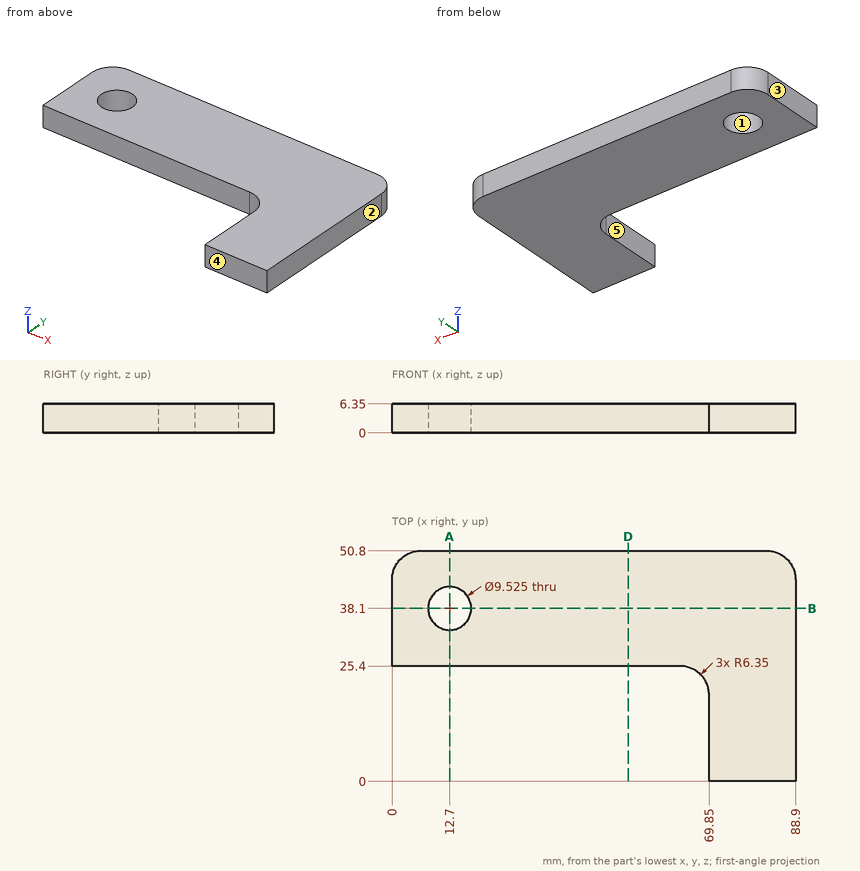
For this review, use the dimensioned drawing (mm, ordinates from the lowest corner) and the shaded views. A direction names the side the tool comes from. Give positions to 0.01 mm unless a question says otherwise; leave off trailing zeros. Loops run counter-clockwise (first coordinate to the right, second up) from the corner with the lowest first, then second, coordinate; pieces in that order, holes last. Notation, with made-up numbers: (-2, 36) -> (23, 36) arc R18 ccw to (23, 52) -> close; hole circle Ø7 at (64.25, 31.5). An arc over 180 degrees is marked (long way). One line per question, with ' | ' between items. Start each with the question number.
(1) For the marked faces 4 and 5, list the 3-axis set-ups (+Z, -Z, +X, -X, +Y, -Y) from which the entire face can be reached by the end or side of a thin tool; tool diameter is ignored.
(2) We need section D-D (x = 52). State the section outline as (y, z) points.
(3) Draft analysis for pull direction X (two halves, no side actions). For the marked faces 1, 2 and 3, state which applies: +X half, -X half, draft (parallel to the pull), parting line (faces both ways), or undercut.
(4) We need section B-B (y = 38.1). State the section outline as (x, z) points, and give its area (3 significant figures).
(5) For line 1 (Y direction, x = 12.7, z = 3.25); line 2 (Y direction, x = 49.5, z = 2.25); line 3 (X direction, y = 39.5, z = 1), list the stretches that pass through material, from the lowest coordinate up.
(6) We need section A-A (x = 12.7). State the section outline as (y, z) points.
(7) Insertion check: P1, Ø8.5, axis at x = 12.7, y = 38.1, coming from the +Z side; P2, Ø1.5, axis at x = 10.5, z = 5, coming from the -Y side. Each pin has a flat end and moves straight along its axis. Give the tip position at first contact, or say it passes through.
The answers:
1) face 4: +Z, -Z, +X, -X, -Y | face 5: +Z, -Z, -X, -Y
2) outline: (25.4, 0) -> (50.8, 0) -> (50.8, 6.35) -> (25.4, 6.35) -> close
3) face 1: undercut | face 2: +X half | face 3: -X half
4) outline: (0, 0) -> (7.94, 0) -> (7.94, 6.35) -> (0, 6.35) -> close; (17.46, 0) -> (88.9, 0) -> (88.9, 6.35) -> (17.46, 6.35) -> close | area: 504 mm^2
5) line 1: y = 25.4 to 33.34, 42.86 to 50.8 | line 2: y = 25.4 to 50.8 | line 3: x = 0 to 8.15, 17.25 to 88.9
6) outline: (25.4, 0) -> (33.34, 0) -> (33.34, 6.35) -> (25.4, 6.35) -> close; (42.86, 0) -> (50.8, 0) -> (50.8, 6.35) -> (42.86, 6.35) -> close
7) P1: passes through | P2: stops at y = 25.4
